Can you work these out from the drawing? Everything is in mm from the part's minimum corner. A direction names the side the tool comes from. Round coordinates to 2 decimals unless told otherwise and drop trailing zeros. Write each loop counter-clockwise with the first axis right and the second up, starting at its lowest first coordinate (ties: lowest second). Pieces come first, ordered by that corner, then holes. Notation, with made-up numbers: (13.25, -30) - (49.25, -30) arc R7 cw to (49.25, -24) - close; hole circle Ø3 at (5.5, 87). An arc over 180 degrees is marked (long way). One line per item, written item: value. Start each with the question number.
Item 1: For P1, Ø6, axis at x = 6, z = 1.5, coming from the +Y side; P2, Ø3, axis at y = 2, z = 9.5, coming from the -X side; P3, Ø2, axis at y = 10, z = 4.5, coming from the +X side; P4, Ø5, axis at x = 10.5, y = 11, coming from the +Z side, each with a flat end and sliding along its axis, tell me the tip position at first contact or that it passes through.
Item 2: Imagine slicing it at C-C, the plane y = 10. Please give me the cut outline in (x, z), then the cut area to 3 significant figures.
Item 3: If I drill on line 1 (X direction, y = 10.25, z = 7); line 2 (Y direction, x = 12.5, z = 7); line 3 (X direction, y = 1.75, z = 7.5), over which ranges is the centre line in solid material (lowest first)?
Item 4: For the marked faces 1 and 2, which set-ups out of +Z, -Z, +X, -X, +Y, -Y let a thin tool reach every point of the face, with its end or its side?
Item 5: Imagine slicing it at D-D, the plane y = 1.25. Please give me the cut outline in (x, z).
Item 6: Imagine slicing it at B-B, the plane z = 7. Please give me the cut outline in (x, y).
Item 7: Imagine slicing it at A-A, the plane x = 7. Please give me the cut outline in (y, z).
Item 8: Thinking about a two-plate mould opening in Z: for the marked faces 3, 4 and 5, which applies, released by +Z, released by -Z, zero draft, split by the parting line, or undercut?
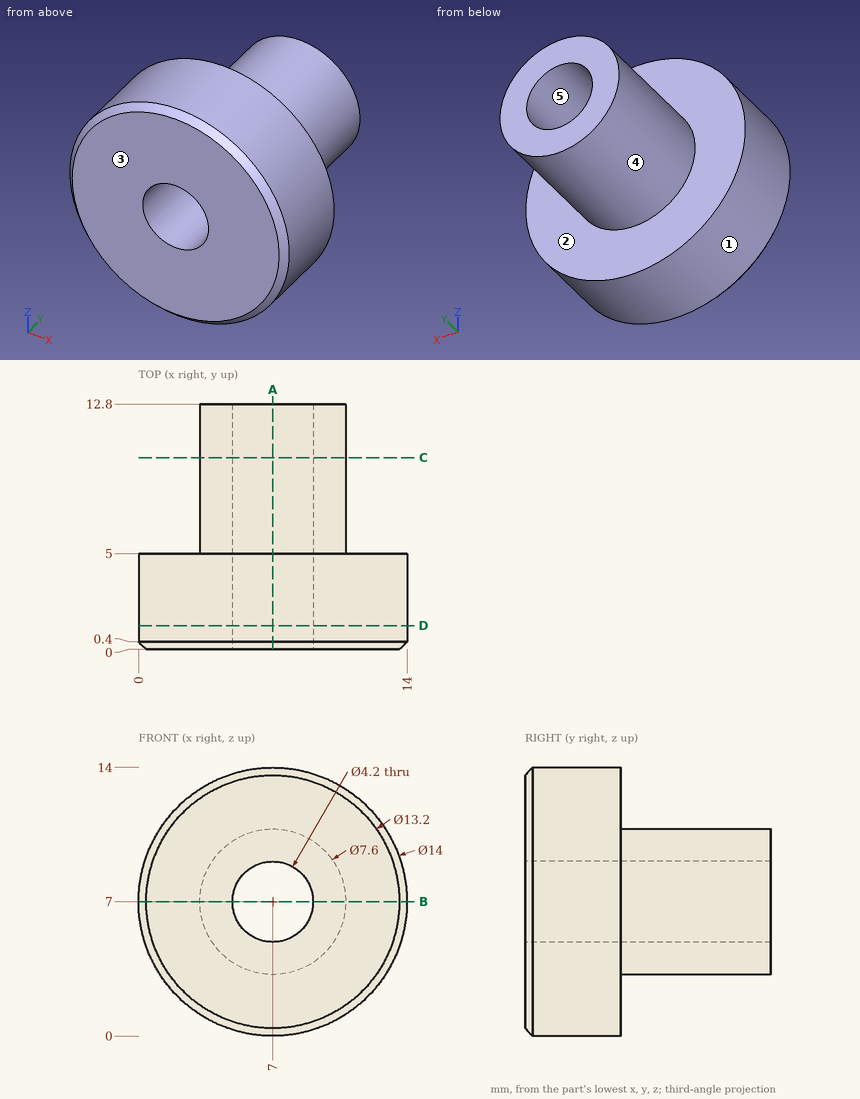
Values follow:
1. P1: stops at y = 12.8
1. P2: stops at x = 0.07
1. P3: stops at x = 10.49
1. P4: stops at z = 10.67
2. outline: circle Ø7.6 at (7, 7); hole circle Ø4.2 at (7, 7)
2. area: 31.5 mm^2
3. line 1: x = 3.2 to 4.9, 9.1 to 10.8
3. line 2: y = 0 to 5
3. line 3: x = 0.02 to 4.96, 9.04 to 13.98
4. face 1: +Y, -Y
4. face 2: +Y
5. outline: circle Ø14 at (7, 7); hole circle Ø4.2 at (7, 7)
6. outline: (0, 0.4) - (0.4, 0) - (4.9, 0) - (4.9, 12.8) - (3.2, 12.8) - (3.2, 5) - (0, 5) - close; (9.1, 0) - (13.6, 0) - (14, 0.4) - (14, 5) - (10.8, 5) - (10.8, 12.8) - (9.1, 12.8) - close
7. outline: (0, 0.4) - (0.4, 0) - (5, 0) - (5, 3.2) - (12.8, 3.2) - (12.8, 4.9) - (0, 4.9) - close; (0, 9.1) - (12.8, 9.1) - (12.8, 10.8) - (5, 10.8) - (5, 14) - (0.4, 14) - (0, 13.6) - close
8. face 3: zero draft
8. face 4: split by the parting line
8. face 5: undercut
